Part print with two shaded views. Sizes in mm from the minimum x, y, z corner. Round coordinates to 2 decimals unless told otherwise and drop trailing zeros. Loops run counter-clockwise (first coordinate to the right, second up) from the corner with the lowest first, then second, coordinate; pieces in that order, holes last.
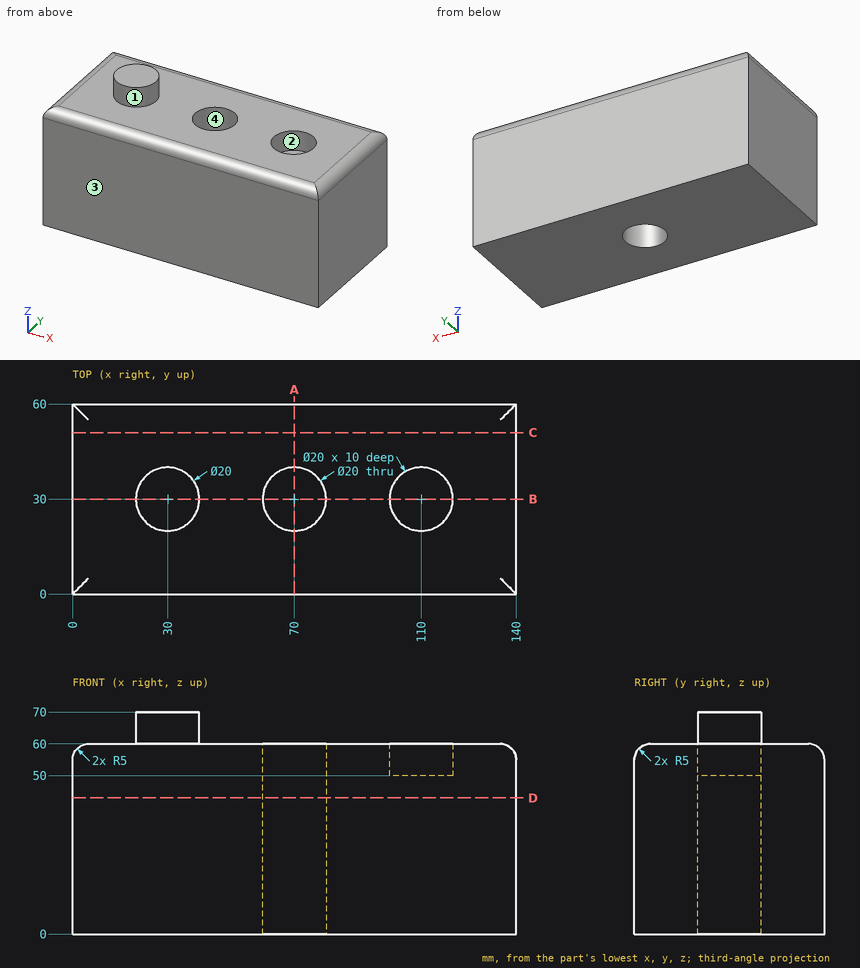
Item 1: Cut at D-D (z = 43). List the corners of the cut face in (x, y).
Verdict:
outline: (0, 0) - (140, 0) - (140, 60) - (0, 60) - close; hole circle Ø20 at (70, 30)
Item 2: Mould opens along Y. For the marked faces 1, 2, 3 and 4 say: released by +Y, released by -Y, zero draft, split by the parting line, or undercut.
Verdict:
face 1: split by the parting line
face 2: undercut
face 3: released by -Y
face 4: undercut
Item 3: Wall check: L1, parallel to Y at x = 110, z = 52; L2, parallel to Y at x = 110, z = 58; L3, parallel to Z at x = 89.5, y = 23. Give the ranges that are in metal, low to high.
Verdict:
L1: y = 0 to 20, 40 to 60
L2: y = 1 to 20, 40 to 59
L3: z = 0 to 60
Item 4: Cut at C-C (y = 51). List the corners of the cut face in (x, z), plus the area to 3 significant figures.
Verdict:
outline: (0, 0) - (140, 0) - (140, 55) arc R5 ccw to (135, 60) - (5, 60) arc R5 ccw to (0, 55) - close
area: 8,390 mm2
Item 5: Flat gauge pins, fed straight in: P1, Ø3, axis at x = 51, y = 47, coming from the -Z side; P2, Ø10, axis at x = 112.5, y = 31, coming from the +Z side; P3, Ø10, axis at x = 37.5, y = 12, coming from the +Z side; P4, Ø2, axis at x = 52.5, z = 57, coming from the +Y side. Where does each tip first touch, or does it go through?
Verdict:
P1: stops at z = 0
P2: stops at z = 50
P3: stops at z = 60
P4: stops at y = 59.9
Item 6: Cut at B-B (y = 30). List the corners of the cut face in (x, z).
Verdict:
outline: (0, 0) - (60, 0) - (60, 60) - (40, 60) - (40, 70) - (20, 70) - (20, 60) - (5, 60) arc R5 ccw to (0, 55) - close; (80, 0) - (140, 0) - (140, 55) arc R5 ccw to (135, 60) - (120, 60) - (120, 50) - (100, 50) - (100, 60) - (80, 60) - close
Item 7: Cut at A-A (x = 70). List the corners of the cut face in (y, z).
Verdict:
outline: (0, 0) - (20, 0) - (20, 60) - (5, 60) arc R5 ccw to (0, 55) - close; (40, 0) - (60, 0) - (60, 55) arc R5 ccw to (55, 60) - (40, 60) - close
